For this review, take the finished solid that the model builds, in its own axes (mm). Face numbers are marked on the shaded views. A direction names the side the tool comes from. Give positions to 0.01 mm unless a question says otherwise; leave off trailing zeros. Order: outer loops, then holes, each group sorted by start corner. A loop starts at its lowest first (then second) coordinate and runs counter-clockwise, first axis right, second up. Notation, with made-up numbers: (76.5, -32.75) -> (82.5, -32.75) arc R11 ccw to (82.5, -19.75) -> close; hole circle Ø10 at (45.25, -1.5). An arc over 180 degrees is marked (long way). Return JSON: item names as keys, results as strings. Group by question number.
1) For the marked faces 1 and 2, list the 3-axis set-ups (+Z, -Z, +X, -X, +Y, -Y) from which the entire face can be reached by the end or side of a thin tool; tool diameter is ignored.
2) Add section A-A (y = 22). Give the boundary of the cut face in (x, z).
3) Add section B-B (z = 26.5). Give the boundary of the cut face in (x, y).
4) Insertion check: P1, Ø3, axis at y = 9.62, z = 23.6, coming from the -X side; P2, Ø20, axis at x = -32, y = 13.5, coming from the -Z side; P3, Ø12, axis at x = -24.5, z = 24, coming from the -Y side; P4, Ø2, axis at x = -14, z = 25, coming from the -Y side. Each pin has a flat end and moves straight along its axis. Give the tip position at first contact, or say it passes through.
5) The part is to be moulded in two halves that separate along X. For the marked faces 3, 4 and 5, say which applies: released by +X, released by -X, zero draft, split by the parting line, or undercut.
6) To check wall thickness, follow line 1 along X through (y, z) = (13.5, 24.5); line 2 along Z through (x, y) = (-42.5, 22.5); line 3 along Z through (x, y) = (-24.5, 2.5). State the ranges of each line that lie inside material, in increasing order.
7) Add section D-D (x = -16). Give the boundary of the cut face in (y, z).
8) Add section C-C (y = 37.5). Give the boundary of the cut face in (x, z).
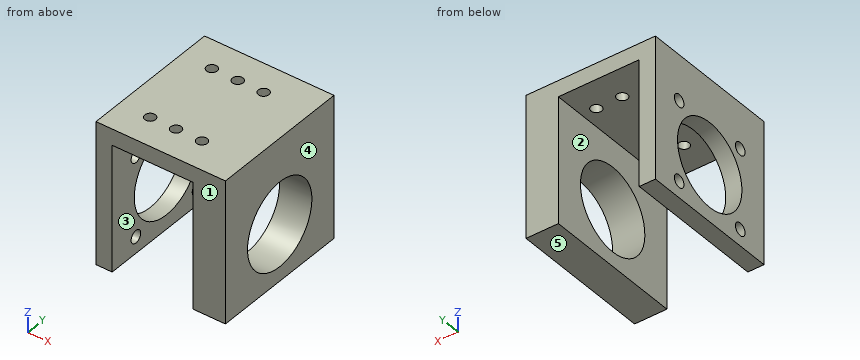
from build123d import *

# Parameters (mm, degrees)
EXTRUDE_1_DEPTH     = 44
SKETCH_3_R          = 1.65
CUT_EXTRUDE_1_DEPTH = 44
SKETCH_6_R          = 1.95
CUT_EXTRUDE_5_DEPTH = 5
SKETCH_4_R          = 13.05
CUT_EXTRUDE_6_DEPTH = 53


with BuildPart() as part:
    # 草图1 → 凸台-拉伸1 (new body)
    with BuildSketch(Plane(origin=(0, 0, 0), x_dir=(1, 0, 0), z_dir=(0, 1, 0))):
        Polygon((-47.233094812, -18.47763864), (-47.233094812, -62.47763864), (-7.233094812, -62.47763864), (-7.233094812, -18.47763864), (-17.233094812, -18.47763864), (-17.233094812, -57.47763864), (-42.233094812, -57.47763864), (-42.233094812, -18.47763864), align=None)
    extrude(amount=EXTRUDE_1_DEPTH)

    # 草图3 → 切除-拉伸1 (cut)
    with BuildSketch(Plane(origin=(0, 0, 57.47763864), x_dir=(-1, 0, 0), z_dir=(0, 0, -1))):
        with Locations((37.733094812, 34.5)):
            Circle(SKETCH_3_R)
        with Locations((37.733094812, 9.5)):
            Circle(SKETCH_3_R)
        with Locations((29.733094812, 34.5)):
            Circle(SKETCH_3_R)
        with Locations((29.733094812, 9.5)):
            Circle(SKETCH_3_R)
        with Locations((21.733094812, 34.5)):
            Circle(SKETCH_3_R)
        with Locations((21.733094812, 9.5)):
            Circle(SKETCH_3_R)
    extrude(amount=-CUT_EXTRUDE_1_DEPTH, mode=Mode.SUBTRACT)

    # 草图6 → 切除-拉伸5 (cut)
    with BuildSketch(Plane.ZY.offset(47.233094812)):
        with Locations((48.34323864, 34.375)):
            Circle(SKETCH_6_R)
        with Locations((23.60323864, 34.375)):
            Circle(SKETCH_6_R)
        with Locations((48.34323864, 9.625)):
            Circle(SKETCH_6_R)
        with Locations((23.60323864, 9.625)):
            Circle(SKETCH_6_R)
    extrude(amount=-CUT_EXTRUDE_5_DEPTH, mode=Mode.SUBTRACT)

    # 草图4 → 切除-拉伸6 (cut)
    with BuildSketch(Plane(origin=(-7.233094812, 0, 0), x_dir=(0, 0, -1), z_dir=(1, 0, 0))):
        with Locations((-35.97763864, 22)):
            Circle(SKETCH_4_R)
    extrude(amount=-CUT_EXTRUDE_6_DEPTH, mode=Mode.SUBTRACT)


solid = part.part
Evaluation:
{
 "1": {"face 1": "+Z, -Z, +X, -X, -Y", "face 2": "-Z, +Y, -Y"},
 "2": {"outline": "(-47.23, 18.48) -> (-42.23, 18.48) -> (-42.23, 22.93) -> (-47.23, 22.93) -> close; (-47.23, 49.03) -> (-42.23, 49.03) -> (-42.23, 57.48) -> (-17.23, 57.48) -> (-17.23, 49.03) -> (-7.23, 49.03) -> (-7.23, 62.48) -> (-47.23, 62.48) -> close; (-17.23, 18.48) -> (-7.23, 18.48) -> (-7.23, 22.93) -> (-17.23, 22.93) -> close"},
 "3": {"outline": "(-47.23, 0) -> (-42.23, 0) -> (-42.23, 13.03) -> (-47.23, 13.03) -> close; (-47.23, 30.97) -> (-42.23, 30.97) -> (-42.23, 44) -> (-47.23, 44) -> close; (-17.23, 0) -> (-7.23, 0) -> (-7.23, 13.03) -> (-17.23, 13.03) -> close; (-17.23, 30.97) -> (-7.23, 30.97) -> (-7.23, 44) -> (-17.23, 44) -> close"},
 "4": {"P1": "x = -17.23", "P2": "z = 57.48", "P3": "through", "P4": "y = 0"},
 "5": {"face 3": "undercut", "face 4": "released by +X", "face 5": "zero draft"},
 "6": {"line 1": "-47.23 to -42.23, -17.23 to -7.23", "line 2": "18.48 to 22.94, 49.02 to 62.48", "line 3": "57.48 to 62.48"},
 "7": {"outline": "(0, 18.48) -> (44, 18.48) -> (44, 62.48) -> (0, 62.48) -> close; hole circle Ø26.1 at (22, 35.98)"},
 "8": {"outline": "(-47.23, 18.48) -> (-42.23, 18.48) -> (-42.23, 57.48) -> (-17.23, 57.48) -> (-17.23, 18.48) -> (-7.23, 18.48) -> (-7.23, 62.48) -> (-47.23, 62.48) -> close"}
}
